Input: part model. Units: mm. Frame: model coordinates. A direction names the side the tool comes from. Give positions to 0.01 mm unless a question says otherwise; leave off trailing zeros. Write each loop counter-clockwise with the first axis right and the second up, starting at its lowest first coordinate (ties: lowest second). Pieces come first, ordered by that corner, then holes. Notation, with made-up numbers: (-15, 45.25) - (28, 45.25) arc R28 cw to (28, 84.25) - close; hole circle Ø3 at (81, -1). An arc over 180 degrees is marked (long way). Use a Markdown table: item, result. Add a question column.
1. Mould query, pull axis X, two halves, no side actions, for faces 1 (the cylindrical face through (-33.476, 33.397, 2.576)), 2 (the flat face through (-24.63, -25.88, 1.25)), 3 (the cylindrical face through (33.476, 33.397, 2.576)). Classes: released by +X, released by -X, zero draft, split by the parting line, or undercut.
2. Section query A-A, the plane y = 0. Return loops of the section in (x, z) (1 decimal).
3. Pin query (flat end, axial travel): pin 1 (2 mm diameter, centred on x = -23, y = 24, fed in from -Z); pin 2 (1.5 mm diameter, centred on x = -20.5, y = 26, fed in from +Z); pin 3 (5.5 mm diameter, centred on x = -24, y = -22, fed in from -Z); pin 4 (8 mm diameter, centred on x = 12.5, y = -18.5, fed in from +Z). Return the tip coordinate at first contact, or that it passes through.
4. Section query B-B, the plane z = 0.95. Count the separate pieces of the cut face and the enclosed holes in it, plus the area to 3 significant figures.
5. Set-up query: faces 4 (the flat face through (0, -28.575, 4)), 5 (the flat face through (26.307, 23, 1)), 6 (the flat face through (0, -34.925, 3)). Return all of +Z, -Z, +X, -X, +Y, -Y with unobstructed straight access to the full face (end or side cutting, diameter ignored); none if empty.
6. Section query C-C, the plane x = 12. Return loops of the section in (y, z) (1 decimal), plus the area to 3 significant figures.
7. Material intervals for probe 1 along X at (y, z) = (11.5, 4.45) (3 decimals); probe 2 along Y at (x, z) = (0, 2.15) (3 decimals), sorted ascending.
```python
from build123d import *

# Parameters (mm, degrees)
F0_W             = 69.85
F0_H             = 69.85
F1_DEPTH         = 5.08
F2_R             = 5.08
F3_R             = 27.78125
F4_DEPTH         = 5.08
F5_W             = 57.15
F5_H             = 57.15
F6_DEPTH         = 1.5875
F8_DEPTH         = 3.4925
F8_COPIES_COUNT  = 4
F11_DEPTH        = 2.54
F11_COPIES_COUNT = 4


# Not quite as in the source:
# - a pattern or mirror of a feature is missing from the dataset's text; its kind, count and spacing are read off the source's solid


with BuildPart() as f1:
    # F0 (on Top) → F1 (new body)
    with BuildSketch(Plane.XY):
        Rectangle(F0_W, F0_H)
    extrude(amount=F1_DEPTH)

    # F2
    f2_edges = [f1.edges().sort_by_distance(p)[0] for p in [
        (-34.925, -34.925, 2.54),
        (34.925, -34.925, 2.54),
        (34.925, 34.925, 2.54),
        (-34.925, 34.925, 2.54),
    ]]
    fillet(f2_edges, radius=F2_R)

    # F3 (on face) → F4 (cut, through all)
    with BuildSketch(Plane.XY.offset(5.08)):
        Circle(F3_R)
    extrude(amount=-F4_DEPTH, mode=Mode.SUBTRACT)

    # F5 (on face) → F6 (cut)
    with BuildSketch(Plane.XY.offset(5.08)):
        Rectangle(F5_W, F5_H)
    extrude(amount=-F6_DEPTH, mode=Mode.SUBTRACT)

    # F7 (on face) → F8 (cut, through all)
    with BuildSketch(Plane.XY.offset(3.4925)):
        with BuildLine():
            Line((21.6602027868, 21.6602027868), (24.3542796231, 24.3542796231))
            ThreePointArc((24.3542796231, 24.3542796231), (21.6602027868, 24.3542796231), (21.6602027868, 21.6602027868))
        make_face()
        with BuildLine():
            ThreePointArc((24.9122412049, 23.0072412049), (24.7672317144, 23.7362531436), (24.3542796231, 24.3542796231))
            Line((24.3542796231, 24.3542796231), (21.6602027868, 21.6602027868))
            ThreePointArc((21.6602027868, 21.6602027868), (23.7362531436, 21.2472506955), (24.9122412049, 23.0072412049))
        make_face()
    f8 = extrude(amount=-F8_DEPTH, mode=Mode.SUBTRACT)

    # F8_copies: F8 ×4 about axis
    f8_copies_axis = Axis((0, 0, 0), (0, 0, 1))
    for i in range(1, F8_COPIES_COUNT):
        add(f8.rotate(f8_copies_axis, i * 360 / F8_COPIES_COUNT), mode=Mode.SUBTRACT)

    # F10 (on face) → F11 (cut)
    with BuildSketch(Plane(origin=(0, 0, 0), x_dir=(1, 0, 0), z_dir=(0, 0, -1))):
        Polygon((26.8172412049, 23.0072412049), (24.9122412049, 26.3067979934), (21.1022412049, 26.3067979934), (19.1972412049, 23.0072412049), (21.1022412049, 19.7076844165), (24.9122412049, 19.7076844165), align=None)
    f11 = extrude(amount=-F11_DEPTH, mode=Mode.SUBTRACT)

    # F11_copies: F11 ×4 about axis
    f11_copies_axis = Axis((0, 0, 0), (0, 0, 1))
    for i in range(1, F11_COPIES_COUNT):
        add(f11.rotate(f11_copies_axis, i * 360 / F11_COPIES_COUNT), mode=Mode.SUBTRACT)


solid = f1.part
```
Result sheet:
| question | item | result |
|---|---|---|
| 1 | face 1 | released by -X |
| 1 | face 2 | undercut |
| 1 | face 3 | released by +X |
| 2 | outline | (-34.9, 0) - (-27.8, 0) - (-27.8, 3.5) - (-28.6, 3.5) - (-28.6, 5.1) - (-34.9, 5.1) - close; (27.8, 0) - (34.9, 0) - (34.9, 5.1) - (28.6, 5.1) - (28.6, 3.5) - (27.8, 3.5) - close |
| 3 | pin 1 | stops at z = 2.54 |
| 3 | pin 2 | stops at z = 3.49 |
| 3 | pin 3 | stops at z = 0 |
| 3 | pin 4 | passes through |
| 4 | separate pieces | 1 |
| 4 | enclosed holes | 5 |
| 4 | area | 2,280 mm² |
| 5 | face 4 | +Z |
| 5 | face 5 | -Z |
| 5 | face 6 | +Z, -Z, +X, -X, -Y |
| 6 | outline | (-34.9, 0) - (-25.1, 0) - (-25.1, 3.5) - (-28.6, 3.5) - (-28.6, 5.1) - (-34.9, 5.1) - close; (25.1, 0) - (34.9, 0) - (34.9, 5.1) - (28.6, 5.1) - (28.6, 3.5) - (25.1, 3.5) - close |
| 6 | area | 89.1 mm² |
| 7 | probe 1 | x = -34.925 to -28.575, 28.575 to 34.925 |
| 7 | probe 2 | y = -34.925 to -27.781, 27.781 to 34.925 |
